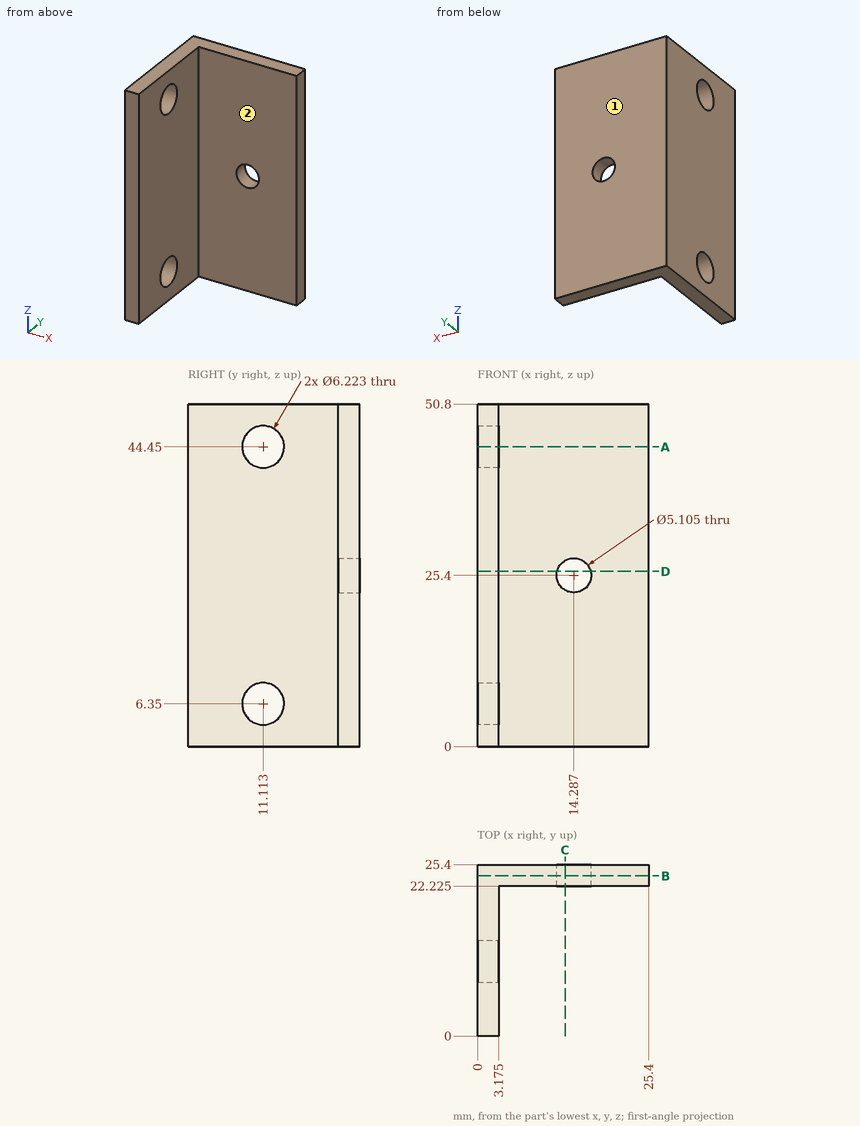
Geometry: see drawing. Coordinates: mm, zero at the bounding-box minimum. A direction names the side the tool comes from. Coordinates: 2 decimals unless noted, no trailing zeros. Order: outer loops, then holes, each group sorted by start corner. A loop starts at its lowest first (then second) coordinate and runs counter-clockwise, first axis right, second up. Notation, with made-up numbers: M 30.25,77.25 L 84.25,77.25 A16 cw 84.25,105.25 Z; hole C -30,-15.5 d6. An arc over 180 degrees is marked long. Answer in a Markdown table with one row per item. Add a question column.
Q1. Section query B-B on y = 23.75. Return the cut outline in (x, z) (1 decimal), and give its area (3 significant figures).
Q2. Section query A-A on z = 44.45. Return the cut outline in (x, y) (1 decimal).
Q3. Reachability of the marked faces 1 and 2 from +Z, -Z, +X, -X, +Y, -Y: full face, straight path, thin tool, end or side. Return the list, or none.
Q4. Line query: L1, parallel to Y at x = 2.1, z = 6.35 (1 decimal); L2, parallel to X at y = 17, z = 46 (1 decimal); L3, parallel to Y at x = 7, z = 5 (1 decimal). Output: solid intervals per line, ascending.
Q5. Contact query for flat-ended pins moving along their axis: P1, Ø6, axis at y = 9.5, z = 20.5, coming from the -X side; P2, Ø11, axis at y = 13.5, z = 13.5, coming from the +X side (1 decimal); P3, Ø2, axis at x = 7.5, z = 13.5, coming from the -Y side (1 decimal); P4, Ø3.5, axis at y = 11.11, z = 44.45, coming from the +X side. Output: stop coordinate, or through.
Q6. Section query D-D on z = 26. Return the cut outline in (x, y) (1 decimal).
Q7. Section query C-C on x = 13. Return the cut outline in (y, z) (1 decimal), and give its area (3 significant figures).
Completed:
| question | item | result |
|---|---|---|
| 1 | outline | M 0,0 L 25.4,0 L 25.4,50.8 L 0,50.8 Z; hole C 14.3,25.4 d5.1 |
| 1 | area | 1,270 mm2 |
| 2 | outline | M 0,0 L 3.2,0 L 3.2,8 L 0,8 Z; M 0,14.2 L 3.2,14.2 L 3.2,22.2 L 25.4,22.2 L 25.4,25.4 L 0,25.4 Z |
| 3 | face 1 | +Z, -Z, +X, -X, +Y |
| 3 | face 2 | +Z, -Z, +X, -Y |
| 4 | L1 | y = 0 to 8, 14.2 to 25.4 |
| 4 | L2 | x = 0 to 3.2 |
| 4 | L3 | y = 22.2 to 25.4 |
| 5 | P1 | stops at x = 0 |
| 5 | P2 | stops at x = 3.2 |
| 5 | P3 | stops at y = 22.2 |
| 5 | P4 | passes through |
| 6 | outline | M 0,0 L 3.2,0 L 3.2,22.2 L 11.8,22.2 L 11.8,25.4 L 0,25.4 Z; M 16.8,22.2 L 25.4,22.2 L 25.4,25.4 L 16.8,25.4 Z |
| 7 | outline | M 22.2,0 L 25.4,0 L 25.4,23.2 L 22.2,23.2 Z; M 22.2,27.6 L 25.4,27.6 L 25.4,50.8 L 22.2,50.8 Z |
| 7 | area | 147 mm2 |
